Here's how the part is built. I have some questions about the finished solid (model axes, mm). Face numbers are marked on the shaded views. Round coordinates to 2 decimals unless told otherwise and drop trailing zeros. Loops run counter-clockwise (first coordinate to the right, second up) from the corner with the lowest first, then second, coordinate; pieces in that order, holes last. Notation, with made-up numbers: M 39,64.5 L 76,64.5 A4 ccw 76,69.5 Z; hole C 27,-5 d4. An arc over 180 degrees is marked long. Use a Markdown table: item, result.
from build123d import *

# Parameters (mm, degrees)
RESSALTO_EXTRUS_O1_DEPTH = 3
ESBO_O2_W                = 47.384173958
ESBO_O2_H                = 2
RESSALTO_EXTRUS_O2_DEPTH = 3
RESSALTO_EXTRUS_O3_DEPTH = 2
RESSALTO_EXTRUS_O5_DEPTH = 12
CORTE_EXTRUS_O1_DEPTH    = 131
CORTE_EXTRUS_O3_DEPTH    = 10


with BuildPart() as part:
    # Esboço1 → Ressalto-extrusão1 (new body)
    with BuildSketch(Plane(origin=(0, 0, 0), x_dir=(1, 0, 0), z_dir=(0, 1, 0))):
        Polygon((53.693575035, 0), (26.846787517, 46.5), (-26.846787517, 46.5), (-53.693575035, 0), (-26.846787517, -46.5), (26.846787517, -46.5), align=None)
    extrude(amount=RESSALTO_EXTRUS_O1_DEPTH)

    # Esboço2 → Ressalto-extrusão2 (add)
    with BuildSketch(Plane(origin=(0, 3, 0), x_dir=(1, 0, 0), z_dir=(0, 1, 0))):
        with Locations((0, 43.5)):
            Rectangle(ESBO_O2_W, ESBO_O2_H)
        Polygon((-50.384173958, -1.732050808), (-26.692086979, -42.767949192), (-24.960036171, -41.767949192), (-48.65212315, -0.732050808), align=None)
        Polygon((26.692086979, -42.767949192), (50.384173958, -1.732050808), (48.65212315, -0.732050808), (24.960036171, -41.767949192), align=None)
    extrude(amount=RESSALTO_EXTRUS_O2_DEPTH)

    # Esboço3 → Ressalto-extrusão3 (add)
    with BuildSketch(Plane.XZ):
        Polygon((26.846787517, 46.5), (-26.846787517, 46.5), (-53.693575035, 0), (-26.846787517, -46.5), (26.846787517, -46.5), (53.693575035, 0), align=None)
    extrude(amount=RESSALTO_EXTRUS_O3_DEPTH)

    # Esboço5 → Ressalto-extrusão5 (add)
    with BuildSketch(Plane.XZ.offset(2)):
        with BuildLine():
            Line((38, 49.00146682), (38, -77.5))
            ThreePointArc((38, -77.5), (36.828427125, -80.328427125), (34, -81.5))
            Line((34, -81.5), (-34, -81.5))
            ThreePointArc((-34, -81.5), (-36.828427125, -80.328427125), (-38, -77.5))
            Line((-38, -77.5), (-38, 49.00146682))
            ThreePointArc((-38, 49.00146682), (-36.828427125, 51.829893945), (-34, 53.00146682))
            Line((-34, 53.00146682), (34, 53.00146682))
            ThreePointArc((34, 53.00146682), (36.828427125, 51.829893945), (38, 49.00146682))
        make_face()
    extrude(amount=RESSALTO_EXTRUS_O5_DEPTH)

    # Esboço7 → Corte-extrusão1 (cut)
    with BuildSketch(Plane(origin=(0, 0, -81.5), x_dir=(-1, 0, 0), z_dir=(0, 0, -1))):
        Polygon((-34.2, -3), (34.2, -3), (34.2, -12.3), (31.2, -12.3), (31.2, -23.281359025), (-31.2, -26.250413902), (-31.2, -12.3), (-34.2, -12.3), align=None)
    extrude(amount=-CORTE_EXTRUS_O1_DEPTH, mode=Mode.SUBTRACT)

    # Esboço8 → Corte-extrusão3 (cut)
    with BuildSketch(Plane.XZ.offset(2)):
        Polygon((-48.693575035, 0), (-38, 0), (-38, -18.521815275), align=None)
        Polygon((38, 0), (48.693575035, 0), (38, -18.521815275), align=None)
    extrude(amount=-CORTE_EXTRUS_O3_DEPTH, mode=Mode.SUBTRACT)


solid = part.part
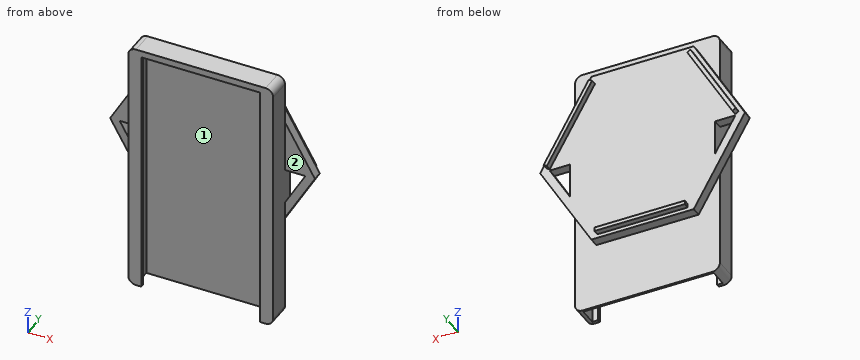
1. Imagine slicing it at D-D, the plane y = -7.25. Write out the boundary of the cut face in (x, z) (3 decimals).
Answer sheet:
| item | result |
|---|---|
| outline | M -38,-77.5 A4 ccw -34.2,-81.495 L -34.2,49.5 L 34.2,49.5 L 34.2,-81.495 A4 ccw 38,-77.5 L 38,49.001 A4 ccw 34,53.001 L -34,53.001 A4 ccw -38,49.001 Z |
2. Imagine slicing it at B-B, the plane z = -57.5. Write out the boundary of the cut face in (x, y), then the cut area to 3 significant figures.
Answer sheet:
| item | result |
|---|---|
| outline | M -38,-14 L -31.2,-14 L -31.2,-12.3 L -34.2,-12.3 L -34.2,-3 L 34.2,-3 L 34.2,-12.3 L 31.2,-12.3 L 31.2,-14 L 38,-14 L 38,-2 L -38,-2 Z |
| area | 170 mm2 |
3. Imagine slicing it at C-C, the plane x = 5. Write out the boundary of the cut face in (y, z), then the cut area to 3 significant figures.
Answer sheet:
| item | result |
|---|---|
| outline | M -14,49.5 L -3,49.5 L -3,-81.5 L -2,-81.5 L -2,-46.5 L 3,-46.5 L 3,-44.5 L 6,-44.5 L 6,-42.5 L 3,-42.5 L 3,46.5 L -2,46.5 L -2,53 L -14,53 Z |
| area | 644 mm2 |
4. We'd pull the mould along X, two halves only. Please class the marked faces 1 and 2: +X half, -X half, draft (parallel to the pull), parting line (faces both ways), or undercut.
Answer sheet:
| item | result |
|---|---|
| face 1 | undercut |
| face 2 | draft |
5. For pin 1 Ø1.5 at (y, z) = (-10.5, 19) entering from +X; pin 2 Ø5.5 at (x, y) = (45, 0) entering from -Z; pin 3 Ø2 at (y, z) = (5, -43) entering from -X; pin 4 Ø5 at (x, y) = (-12.5, -1) entering from -Z, each with a flat end and sliding along its axis, tell me the tip position at first contact or that it passes through.
Answer sheet:
| item | result |
|---|---|
| pin 1 | x = 38 |
| pin 2 | z = -19.82 |
| pin 3 | x = -23.69 |
| pin 4 | z = -81.5 |
6. I need wall thicknesses on probe 1 along X at (y, z) = (-4.75, 23.5); probe 2 along X at (y, z) = (-13, -62); probe 3 along X at (y, z) = (-2.25, -23.5). Which ranges of each line are inside material? Lowest first, please. Write a range as from..to.
Answer sheet:
| item | result |
|---|---|
| probe 1 | -38..-34.2, 34.2..38 |
| probe 2 | -38..-31.2, 31.2..38 |
| probe 3 | -38..38 |
7. Imagine slicing it at A-A, the plane y = 1.25. Write out the boundary of the cut face in (x, z), then the cut area to 3 significant figures.
Answer sheet:
| item | result |
|---|---|
| outline | M -53.69,0 L -26.85,-46.5 L 26.85,-46.5 L 53.69,0 L 26.85,46.5 L -26.85,46.5 Z; hole M -48.69,0 L -38,-18.52 L -38,0 Z; hole M 38,-18.52 L 48.69,0 L 38,0 Z |
| area | 7,290 mm2 |
